CAD build for the part. Positions are in the model's coordinates, mm. Face numbers are marked on the shaded views. A direction names the side the tool comes from. Coordinates: 2 decimals unless noted, no trailing zeros. Loops run counter-clockwise (first coordinate to the right, second up) from the corner with the lowest first, then second, coordinate; pieces in that order, holes last. Notation, with made-up numbers: M 6,59 L 52,59 A19 cw 52,75 Z; hole C -10.5,-16 d5. An arc over 180 degrees is marked long. Answer as a JSON object with one key per item and string values. Group by question number.
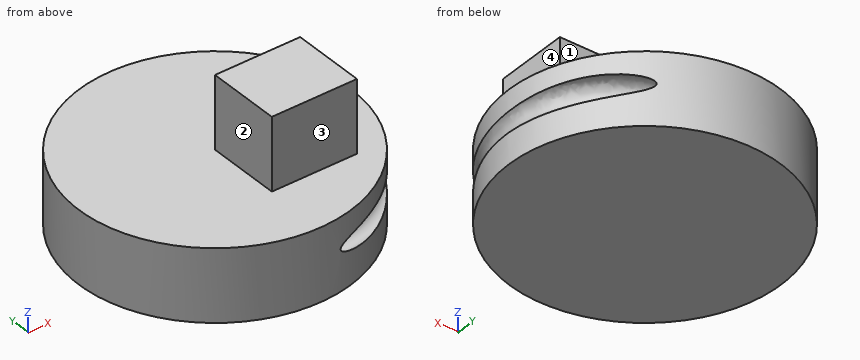
```python
from build123d import *

# Parameters (mm, degrees)
F1_R     = 47.8906341697
F3_DEPTH = 25.4
F2_W     = 30.0199426711
F2_H     = 25.7944688201
F4_DEPTH = 25.4
F7_R     = 4.2429445986


# Not quite as in the source:
# - a feature of the source that left no trace in its solid (it failed there, or was rolled back) is left out


with BuildPart() as f3:
    # F1 (on Top) → F3 (new body)
    with BuildSketch(Plane.XY):
        Circle(F1_R)
    extrude(amount=F3_DEPTH)

    # F2 (on offset) → F4 (join)
    with BuildSketch(Plane.XY.offset(50.8)):
        with Locations((15.0099713355, -12.89723441)):
            Rectangle(F2_W, F2_H)
    extrude(amount=-F4_DEPTH)

    # F8: sweep along a path in F6
    with BuildLine(Plane.XY.offset(12.7)) as f8_path:
        CenterArc((9.0787773952, -2.0044676494), 44.2959341801, 0, 360)
    # F7 (on Front) → F8 (sweep, cut)
    with BuildSketch(Plane.XZ):
        with Locations((50.1028448343, 14.4018204883)):
            Circle(F7_R)
    sweep(path=f8_path.line, mode=Mode.SUBTRACT)


solid = f3.part
```
Item 1: Slice it at C-C, the plane z = 29. Write the cut outline in (x, y), then the cut area to 3 significant figures.
Item 2: Tool access for the marked faces 1, 2, 3 and 4: list every direction of +Z, -Z, +X, -X, +Y, -Y with a clear straight run to the whole face (end or side of a thin tool).
Item 3: Slice it at B-B, the plane x = -15.5. Count the separate pieces of the cut face and the enclosed holes in it, then the cut area to 3 significant figures.
Item 4: Slice it at A-A, the plane z = 20. Write the cut outline in (x, y).
Item 5: Drill centre lines: L1, parallel to Y at x = -11, z = 15.5; L2, parallel to Y at x = -4, z = 13; L3, parallel to Z at x = -39, y = -7.5. Where is each one in solid material? Low to high. Write a range as from..to.
Item 6: Pin check, flat tips, straight feed: pin 1 (4 mm diameter, centred on x = 14.5, y = 19, fed in from +Z); pin 2 (8 mm diameter, centred on y = 35.5, z = 10, fed in from -X); pin 3 (20.5 mm diameter, centred on y = -8, z = 40.5, fed in from -X). Stop position of each tip, or through.
Computed:
{
 "1": {"outline": "M 0,-25.79 L 30.02,-25.79 L 30.02,0 L 0,0 Z", "area": "774 mm2"},
 "2": {"face 1": "+Z, +X, -X, +Y", "face 2": "+Z, -X, +Y, -Y", "face 3": "+Z, +X, -X, -Y", "face 4": "+Z, +X, +Y, -Y"},
 "3": {"separate pieces": "1", "enclosed holes": "2", "area": "2,160 mm2"},
 "4": {"outline": "C 0,0 d95.78"},
 "5": {"L1": "-46.61..-42.46, -33.06..29.05, 38.45..46.61", "L2": "-47.72..-45.14, -36.69..32.69, 41.13..47.72", "L3": "0..25.4"},
 "6": {"pin 1": "z = 25.4", "pin 2": "x = -36.07", "pin 3": "x = 0"}
}
